Read the model definition and answer for the solid it produces. Units are mm, in the model's axes. Face numbers are marked on the shaded views. A direction names the side the tool comes from. Give positions to 0.01 mm unless a question says otherwise; leave off trailing zeros. Write each loop counter-clockwise with the first axis right and the second up, starting at its lowest first coordinate (ties: lowest second). Pieces come first, ordered by that corner, then holes. Notation, with made-up numbers: M 59,-4 L 96,-4 A25 cw 96,34 Z; hole C 59,-18 d11. An arc over 180 degrees is marked long. Answer as CSV lines item,"result". Start each with the question number.
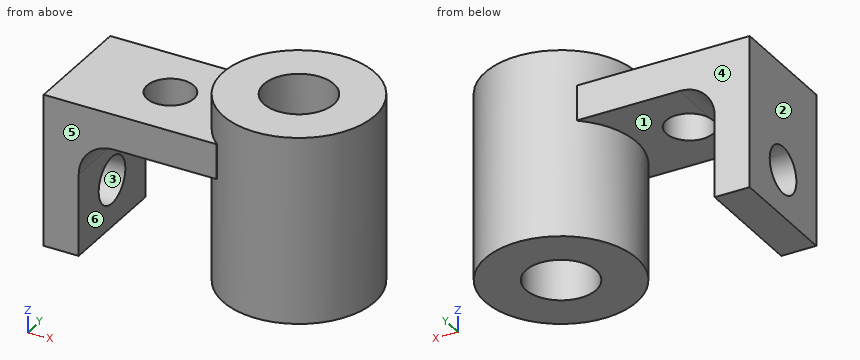
Autodesk Inventor part; units mm, degrees
ref_plane "Płaszczyzna konstrukcyjna2" through (0, 32.5, 0) normal (0, 1, 0) x (-1, 0, 0)
ref_plane "Płaszczyzna konstrukcyjna3" through (0, 16.25, 0) normal (0, 1, 0) x (-1, 0, 0)
ref_plane "YZ Plane" through (0, 0, 0) normal (1, 0, 0) x (0, 1, 0)
sketch "Szkic1" plane through (0, 0, 0) normal (0, 0, 1) x (1, 0, 0)
  circle A0 centre (0, 0) radius 15
  circle A1 centre (0, 0) radius 32.5
  dimension "d0" = 65
  dimension "d1" = 30
extrude "Wyciągnięcie proste1" add sketch "Szkic1" along normal blind 80
sketch "Szkic2" plane through (0, 0, 0) normal (0, 1, 0) x (-1, 0, 0)
  point P0 (0, 0)
ref_plane "Płaszczyzna konstrukcyjna2" through (0, 32.5, 0) normal (0, 1, 0) x (-1, 0, 0)
sketch "Szkic3" plane through (0, 32.5, 0) normal (0, 1, 0) x (-1, 0, 0)
  line L0 (32.5, 80) -> (-32.5, 80)
  line L1 (32.5, 0) -> (-32.5, 0)
  line L2 (32.5, 0) -> (32.5, 80)
  line L3 (32.5, 0) -> (-32.5, 0)
  line L4 (-32.5, 0) -> (-32.5, 80)
  line L5 (21, 65) -> (95, 65)
  line L6 (95, 65) -> (95, 0)
  line L7 (95, 0) -> (80, 0)
  line L8 (80, 0) -> (80, 35)
  line L9 (65, 50) -> (21, 50)
  line L10 (21, 50) -> (21, 65)
  arc A0 (80, 35) -> (65, 50) centre (65, 35) ccw
  line L11 (0, 80) -> (0, 0) construction
  dimension "d4" = 15
  dimension "d8" = 15
  dimension "d10" = 65
  dimension "d11" = 65
  dimension "d12" = 95
  dimension "d15" = 15
ref_plane "Płaszczyzna konstrukcyjna3" through (0, 16.25, 0) normal (0, 1, 0) x (-1, 0, 0)
sketch "Szkic4" plane through (0, 0, 0) normal (0, 1, 0) x (-1, 0, 0)
  line L0 (21, 65) -> (95, 65)
  line L1 (21, 50) -> (21, 65)
  line L2 (65, 50) -> (21, 50)
  arc A0 (80, 35) -> (65, 50) centre (65, 35) ccw
  line L3 (80, 0) -> (80, 35)
  line L4 (95, 65) -> (95, 0)
  line L5 (95, 0) -> (80, 0)
  point P0 (0, 0)
extrude "Wyciągnięcie proste2" add sketch "Szkic4" along normal mid plane 50
sketch "Szkic5" plane through (-95, -25, 65) normal (-1, 0, 0) x (0, 0, 1)
  circle A0 centre (-45, 25) radius 10
  line L0 (-65, 0) -> (-65, 50)
  point P0 (-65, 25)
  dimension "d16" = 20
  dimension "d17" = 20
extrude "Wyciągnięcie proste3" cut sketch "Szkic5" against normal blind 50
sketch "Szkic6" plane through (-95, 25, 65) normal (0, 0, 1) x (1, 0, 0)
  circle A0 centre (40, -25) radius 10
  point P0 (95, -25)
  dimension "d20" = 20
  dimension "d21" = 55
extrude "Wyciągnięcie proste4" cut sketch "Szkic6" against normal blind 50
properties part number "Bartosz_Zukowski_model_nr_10"
1. Given pin 1 (5 mm diameter, centred on x = -13.5, z = 9.5, fed in from +Y); pin 2 (3 mm diameter, centred on x = -8, z = 45.5, fed in from +Y); pin 3 (3 mm diameter, centred on x = -74.5, y = 12, fed in from -Z), each flat-ended and moving along its own axis, determine where each tip first touches the part or whether it passes through.
2. Find section B-B on x = -55. Determine the outline of the cut face in (y, z).
3. Find section D-D on y = 16.5. Determine the outline of the cut face in (x, z).
4. Find the intervals of material crossed by line 1 (Y direction, x = -91.75, z = 20); line 2 (X direction, y = 13, z = 11); line 3 (X direction, y = -10, z = 14.5), in increasing order. Write a range as [from, to].
5. Determine the mould class of the marked faces 1, 2 and 3 for opening direction X: +X half, -X half, draft (parallel to the pull), parting line (faces both ways), or undercut.
6. For the marked faces 4, 5 and 6, determine the directions among +Z, -Z, +X, -X, +Y, -Y from which every point of the face is accessible in a straight line to the end or side of a thin tool.
7. Find section C-C on z = 42. Determine the outline of the cut face in (x, y), then the cut area to 3 significant figures.
8. Find section A-A on z = 20. Determine the outline of the cut face in (x, y).
Computed:
1,pin 1,"stops at y = 30.58"
1,pin 2,"stops at y = 31.84"
1,pin 3,"stops at z = 45.2"
2,outline,"M -25,50 L -10,50 L -10,65 L -25,65 Z; M 10,50 L 25,50 L 25,65 L 10,65 Z"
3,outline,"M -95,0 L -80,0 L -80,35 A15 cw -65,50 L -28,50 L -28,0 L 28,0 L 28,80 L -28,80 L -28,65 L -95,65 Z"
4,line 1,"y = [-25, -10], [10, 25]"
4,line 2,"x = [-95, -80], [-29.79, -7.48], [7.48, 29.79]"
4,line 3,"x = [-95, -80], [-30.92, -11.18], [11.18, 30.92]"
5,face 1,"undercut"
5,face 2,"-X half"
5,face 3,"draft"
6,face 4,"+Z, -Z, -X, +Y"
6,face 5,"+Z, -Z, -X, -Y"
6,face 6,"-Z, +Y, -Y"
7,outline,"M -95,-25 L -78.27,-25 L -78.27,25 L -95,25 Z; C 0,0 d65; hole C 0,0 d30"
7,area,"3,450 mm^2"
8,outline,"M -95,-25 L -80,-25 L -80,-10 L -95,-10 Z; M -95,10 L -80,10 L -80,25 L -95,25 Z; C 0,0 d65; hole C 0,0 d30"
